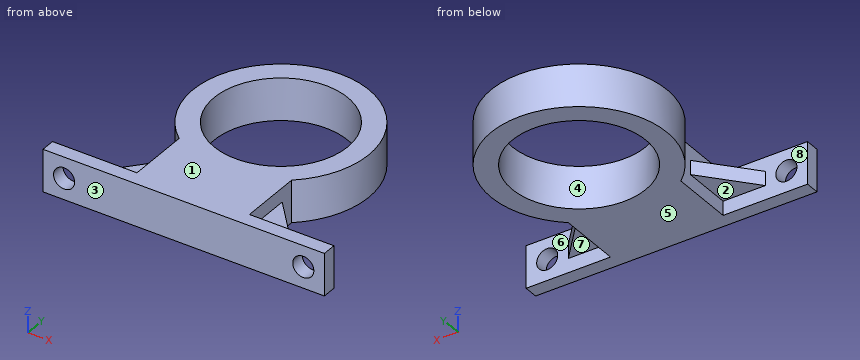
```python
from build123d import *

# Parameters (mm, degrees)
SKETCH1_R                            = 12.5
SKETCH1_R_2                          = 9.5
BOSS_EXTRUDE1_DEPTH                  = 6
SKETCH2_W                            = 16
SKETCH2_H                            = 6
BOSS_EXTRUDE2_DEPTH                  = 8
BOSS_EXTRUDE2_DIRECTION_2_REACH      = 30.588
BOSS_EXTRUDE2_DIRECTION_2_END_RADIUS = 12.5
SKETCH3_W                            = 6
SKETCH3_H                            = 2
BOSS_EXTRUDE3_DEPTH                  = 12
BOSS_EXTRUDE4_DEPTH                  = 1
CUT_EXTRUDE1_REACH                   = 39.376
SKETCH7_R                            = 1.5


with BuildPart() as part:
    # Sketch1 → Boss-Extrude1 (new body)
    with BuildSketch(Plane.XY):
        Circle(SKETCH1_R)
        Circle(SKETCH1_R_2, mode=Mode.SUBTRACT)
    extrude(amount=BOSS_EXTRUDE1_DEPTH)

    # Sketch2 → Boss-Extrude2 (add)
    with BuildSketch(Plane(origin=(0, -12.5, 0), x_dir=(-1, 0, 0), z_dir=(0, -1, 0))):
        with Locations((0, -3)):
            Rectangle(SKETCH2_W, SKETCH2_H)
    extrude(amount=BOSS_EXTRUDE2_DEPTH)

    # Boss-Extrude2 direction 2: up to this cylinder (the profile starts outside it)
    boss_extrude2_direction_2_end = Plane(origin=(0, 0, 3), z_dir=(0, 0, -1)) * Cylinder(BOSS_EXTRUDE2_DIRECTION_2_END_RADIUS, 87.176, mode=Mode.PRIVATE)
    # Sketch2 → Boss-Extrude2 direction 2 (add, up to the surface)
    with BuildSketch(Plane(origin=(0, -12.5, 0), x_dir=(-1, 0, 0), z_dir=(0, -1, 0)), mode=Mode.PRIVATE) as boss_extrude2_direction_2_sk1:
        with Locations((0, -3)):
            Rectangle(SKETCH2_W, SKETCH2_H)
    boss_extrude2_direction_2_tool1 = extrude(boss_extrude2_direction_2_sk1.sketch, amount=-BOSS_EXTRUDE2_DIRECTION_2_REACH, mode=Mode.PRIVATE) - boss_extrude2_direction_2_end
    add(boss_extrude2_direction_2_tool1.solids().sort_by_distance((0, -12.5, 3))[0])
    add(boss_extrude2_direction_2_tool1.solids().sort_by_distance((0, -12.5, 3))[1])

    # Sketch3 → Boss-Extrude3 (add)
    with BuildSketch(Plane(origin=(8, 0, 0), x_dir=(0, 0, -1), z_dir=(1, 0, 0))):
        with Locations((-3, -19.5)):
            Rectangle(SKETCH3_W, SKETCH3_H)
    boss_extrude3 = extrude(amount=BOSS_EXTRUDE3_DEPTH)

    # Mirror1: Boss-Extrude3 across plane
    add(boss_extrude3.mirror(Plane(origin=(0, 0, 0), x_dir=(0, 0, 1), z_dir=(1, 0, 0))))

    # Sketch6 → Boss-Extrude4 (add, symmetric)
    with BuildSketch(Plane.XY.offset(3)):
        Polygon((14, -18.5), (8, -11.604686356), (8, -18.5), align=None)
    boss_extrude4 = extrude(amount=BOSS_EXTRUDE4_DEPTH, both=True)

    # Mirror2: Boss-Extrude4 across plane
    add(boss_extrude4.mirror(Plane(origin=(0, 0, 0), x_dir=(0, 0, 1), z_dir=(1, 0, 0))))

    # Sketch7 → Cut-Extrude1 (cut, up to next)
    with BuildSketch(Plane(origin=(0, -18.5, 0), x_dir=(1, 0, 0), z_dir=(0, 1, 0)), mode=Mode.PRIVATE) as cut_extrude1_sk1:
        with Locations(Location((-17, -3, 0), (0, 0, 270))):
            Circle(SKETCH7_R)
    cut_extrude1_tool1 = extrude(cut_extrude1_sk1.sketch, amount=-CUT_EXTRUDE1_REACH, mode=Mode.PRIVATE) & part.part
    # Sketch7 → Cut-Extrude1 (cut, up to next)
    with BuildSketch(Plane(origin=(0, -18.5, 0), x_dir=(1, 0, 0), z_dir=(0, 1, 0)), mode=Mode.PRIVATE) as cut_extrude1_sk2:
        with Locations(Location((17, -3, 0), (0, 0, 270))):
            Circle(SKETCH7_R)
    cut_extrude1_tool2 = extrude(cut_extrude1_sk2.sketch, amount=-CUT_EXTRUDE1_REACH, mode=Mode.PRIVATE) & part.part
    add(cut_extrude1_tool1.solids().sort_by_distance((-17, -18.5, 3))[0], mode=Mode.SUBTRACT)
    add(cut_extrude1_tool2.solids().sort_by_distance((17, -18.5, 3))[0], mode=Mode.SUBTRACT)


solid = part.part
```
For this review, take the finished solid that the model builds, in its own axes (mm). Face numbers are marked on the shaded views. A direction names the side the tool comes from. Give positions to 0.01 mm unless a question says otherwise; leave off trailing zeros. Write each loop counter-clockwise with the first axis right and the second up, starting at its lowest first coordinate (ties: lowest second). Pieces come first, ordered by that corner, then holes. Notation, with made-up numbers: M 68,-32.75 L 101,-32.75 A16 cw 101,-7.75 Z; hole C 36.5,12 d3. An arc over 180 degrees is marked long. One line per item, written item: value.
1) The part is to be moulded in two halves that separate along Y. For the marked faces 1, 2 and 3, say which applies: +Y half, -Y half, draft (parallel to the pull), parting line (faces both ways), or undercut.
Results are:
face 1: draft
face 2: undercut
face 3: -Y half
2) For P1, Ø4, axis at x = 0, y = 5.5, coming from the +Z side; P2, Ø1, axis at y = -0.5, z = 2.5, coming from the +X side; P3, Ø3, axis at x = -12, y = -16, coming from the +Z side; P4, Ø1, axis at y = -15, z = 4, coming from the +X side, all flat-tipped, find the tip position at first contact; note any pin that passes through.
Results are:
P1: passes through
P2: stops at x = 12.5
P3: stops at z = 4
P4: stops at x = 11.39
3) Take a section at D-D, the plane y = -15. Write out the cut boundary in (x, z), then the cut area to 3 significant figures.
Results are:
outline: M -10.95,2 L -8,2 L -8,0 L 8,0 L 8,2 L 10.95,2 L 10.95,4 L 8,4 L 8,6 L -8,6 L -8,4 L -10.95,4 Z
area: 108 mm²
4) For the marked faces 4, 5, 6, 7 and 8, list the 3-axis set-ups (+Z, -Z, +X, -X, +Y, -Y) from which the entire face can be reached by the end or side of a thin tool; tool diameter is ignored.
Results are:
face 4: +Z, -Z
face 5: -Z, +X, -X, +Y, -Y
face 6: +X
face 7: -Z, +X
face 8: -X
5) For line 1 (X direction, y = -19.8, z = 3); line 2 (Y direction, x = -8.5, z = 1.5); line 3 (Y direction, x = 0, z = 4.05), list the stretches that pass through material, from the lowest coordinate up. Write a range as from..to.
Results are:
line 1: x = -20..-18.5, -15.5..15.5, 18.5..20
line 2: y = -20.5..-18.5, -9.17..-4.24, 4.24..9.17
line 3: y = -20.5..-9.5, 9.5..12.5
6) Take a section at B-B, the plane y = 0. Write out the cut boundary in (x, z).
Results are:
outline: M -12.5,0 L -9.5,0 L -9.5,6 L -12.5,6 Z; M 9.5,0 L 12.5,0 L 12.5,6 L 9.5,6 Z
7) Take a section at C-C, the plane x = -17. Write out the cut boundary in (y, z).
Results are:
outline: M -20.5,0 L -18.5,0 L -18.5,1.5 L -20.5,1.5 Z; M -20.5,4.5 L -18.5,4.5 L -18.5,6 L -20.5,6 Z
8) Take a section at A-A, the plane z = 3. Write out the cut boundary in (x, y).
Results are:
outline: M -20,-20.5 L -18.5,-20.5 L -18.5,-18.5 L -20,-18.5 Z; M -15.5,-20.5 L 15.5,-20.5 L 15.5,-18.5 L 14,-18.5 L 8,-11.6 L 8,-9.6 A12.5 ccw long -8,-9.6 L -8,-11.6 L -14,-18.5 L -15.5,-18.5 Z; M 18.5,-20.5 L 20,-20.5 L 20,-18.5 L 18.5,-18.5 Z; hole C 0,0 d19
